The model under review builds one solid part; all positions refer to its coordinate system, in mm. Give positions to 0.01 mm unless a question says otherwise; leave off trailing zeros. Order: outer loops, then holes, each group sorted by start corner. A loop starts at its lowest first (then second) coordinate and runs counter-clockwise, first axis right, second up. Notation, with made-up numbers: (75, -38) - (95, -38) arc R8 cw to (95, -26) - close; hole circle Ø3 at (39, -13.75). An arc over 180 degrees is marked (long way). Answer as CSV lines item,"result". Start each with the question number.
from build123d import *

# Parameters (mm, degrees)
SKETCH1_R           = 36.15
SKETCH1_R_2         = 2.5
BOSS_EXTRUDE1_DEPTH = 4


with BuildPart() as part:
    # Sketch1 → Boss-Extrude1 (new body)
    with BuildSketch(Plane(origin=(0, 0, 0), x_dir=(1, 0, 0), z_dir=(0, 1, 0))):
        with Locations(Location((0, 0, 0), (0, 0, 270))):
            Circle(SKETCH1_R)
        with Locations(Location((0, 0, 0), (0, 0, 270))):
            Circle(SKETCH1_R_2, mode=Mode.SUBTRACT)
        with BuildLine():
            ThreePointArc((4, -30.892110643), (22.026376234, -22.026376234), (30.892110643, -4))
            Line((30.892110643, -4), (6, -4))
            ThreePointArc((6, -4), (4.585786438, -4.585786438), (4, -6))
            Line((4, -6), (4, -30.892110643))
        make_face(mode=Mode.SUBTRACT)
        with BuildLine():
            ThreePointArc((30.892110643, 4), (22.026376234, 22.026376234), (4, 30.892110643))
            Line((4, 30.892110643), (4, 6))
            ThreePointArc((4, 6), (4.585786438, 4.585786438), (6, 4))
            Line((6, 4), (30.892110643, 4))
        make_face(mode=Mode.SUBTRACT)
        with BuildLine():
            ThreePointArc((-4, 30.892110643), (-22.026376234, 22.026376234), (-30.892110643, 4))
            Line((-30.892110643, 4), (-6, 4))
            ThreePointArc((-6, 4), (-4.585786438, 4.585786438), (-4, 6))
            Line((-4, 6), (-4, 30.892110643))
        make_face(mode=Mode.SUBTRACT)
        with BuildLine():
            Line((-30.892110643, -4), (-6, -4))
            ThreePointArc((-6, -4), (-4.585786438, -4.585786438), (-4, -6))
            Line((-4, -6), (-4, -30.892110643))
            ThreePointArc((-4, -30.892110643), (-22.026376234, -22.026376234), (-30.892110643, -4))
        make_face(mode=Mode.SUBTRACT)
    extrude(amount=BOSS_EXTRUDE1_DEPTH)


solid = part.part
Item 1: Mouldability with a two-part tool opening along Z and no side actions: class faces 1 (the face through (-35.3, 2, -7.8)), 2 (the face through (4.6, 1.97, 4.57)), 3 (the face through (-8, 4, -1)) as released by +Z, released by -Z, zero draft, split by the parting line, or undercut.
Item 2: For line 1 along X through (y, z) = (1.8, 0); line 2 along Z through (x, y) = (-18, 3.1); line 3 along Z through (x, y) = (12.5, 2.6), list the stretches that pass through material, from the lowest coordinate up.
Item 3: Take a section at B-B on z = 0. Write out the cut boundary in (x, y).
Item 4: Take a section at C-C on y = 0.75. Write out the cut boundary in (x, z).
Item 5: Take a section at D-D on x = 14.5. Write out the cut boundary in (y, z).
Item 6: Take a section at A-A on x = 0. Write out the cut boundary in (y, z), and give its area (3 significant figures).
Item 7: Clearance check with flat-ended pins moving along their axes: pin 1 (2 mm diameter, centred on y = 2.5, z = 13, fed in from -X); pin 2 (2 mm diameter, centred on x = -21.5, y = 2, fed in from +Z); pin 3 (1.5 mm diameter, centred on x = 9, y = 1.5, fed in from -Z). State where each tip first meets the part, or that it passes through.
Data:
1,face 1,"split by the parting line"
1,face 2,"undercut"
1,face 3,"zero draft"
2,line 1,"x = -36.15 to -2.5, 2.5 to 36.15"
2,line 2,"z = -31.35 to -25.42, -4 to 4, 25.42 to 31.35"
2,line 3,"z = -33.92 to -28.53, -4 to 4, 28.53 to 33.92"
3,outline,"(-36.15, 0) - (-2.5, 0) - (-2.5, 4) - (-36.15, 4) - close; (2.5, 0) - (36.15, 0) - (36.15, 4) - (2.5, 4) - close"
4,outline,"circle Ø72.3 at (0, 0); hole (-30.89, -4) arc R31.15 ccw to (-4, -30.89) - (-4, -6) arc R2 ccw to (-6, -4) - close; hole (-30.89, 4) - (-6, 4) arc R2 ccw to (-4, 6) - (-4, 30.89) arc R31.15 ccw to start; hole circle Ø5 at (0, 0); hole (4, -30.89) arc R31.15 ccw to (30.89, -4) - (6, -4) arc R2 ccw to (4, -6) - close; hole (4, 6) arc R2 ccw to (6, 4) - (30.89, 4) arc R31.15 ccw to (4, 30.89) - close"
5,outline,"(0, -33.11) - (4, -33.11) - (4, -27.57) - (0, -27.57) - close; (0, -4) - (4, -4) - (4, 4) - (0, 4) - close; (0, 27.57) - (4, 27.57) - (4, 33.11) - (0, 33.11) - close"
6,outline,"(0, -36.15) - (4, -36.15) - (4, -2.5) - (0, -2.5) - close; (0, 2.5) - (4, 2.5) - (4, 36.15) - (0, 36.15) - close"
6,area,"269 mm^2"
7,pin 1,"stops at x = -34.1"
7,pin 2,"stops at z = 29.78"
7,pin 3,"stops at z = -35.2"
